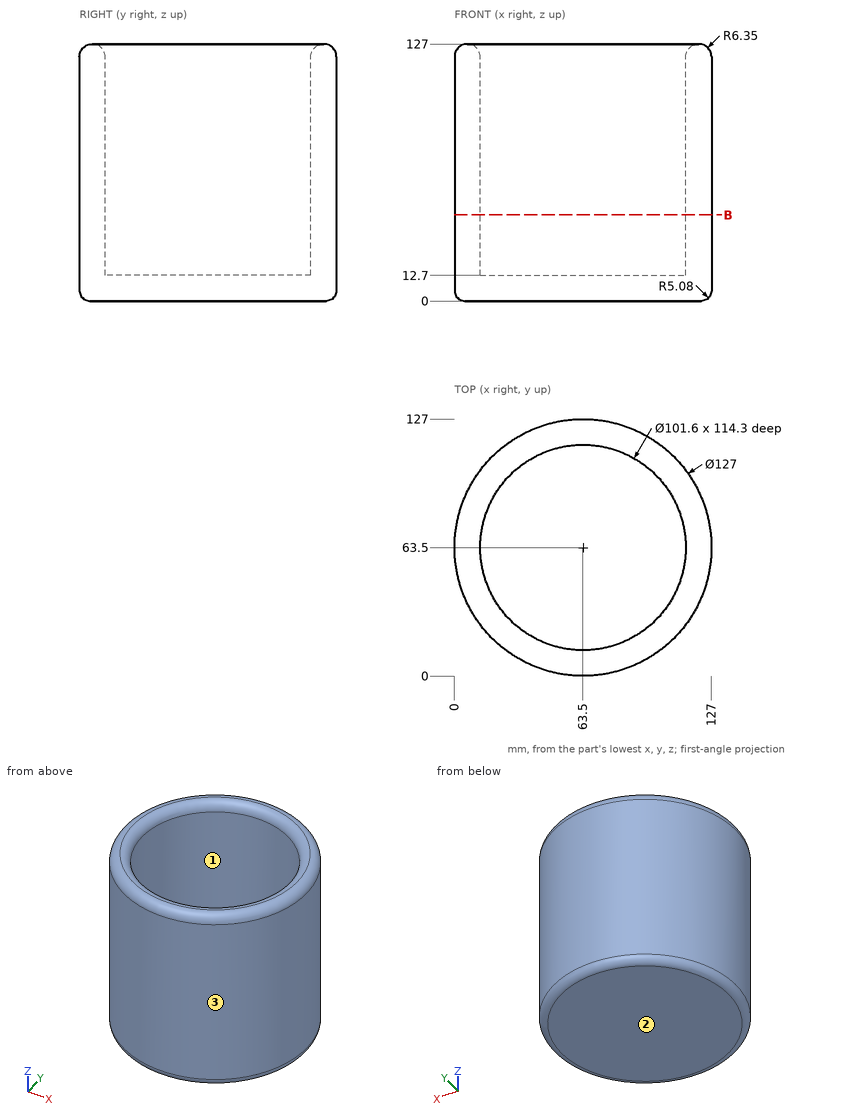
Here's the drawing with two shaded views (mm, measured from the low corner). I have some questions. Round coordinates to 2 decimals unless told otherwise and drop trailing zeros. Loops run counter-clockwise (first coordinate to the right, second up) from the corner with the lowest first, then second, coordinate; pieces in that order, holes last.
Item 1: Please list where these lines run through material, in increasing order: L1, parallel to Y at x = 64.5, z = 72; L2, parallel to X at y = 63, z = 39; L3, parallel to Z at x = 26.5, y = 55.
Item 2: If we mould it in two halves opening along X, with no side actions, what happens to the marked faces 1, 2 and 3? For each: +X half, -X half, draft (parallel to the pull), parting line (faces both ways), or undercut.
Item 3: Will these pins go through, and if not, where does the flat tip stop? pin 1 Ø1 at (y, z) = (32, 67) entering from +X; pin 2 Ø3 at (x, z) = (80.5, 85) entering from -Y; pin 3 Ø8 at (x, y) = (81.5, 45) entering from +Z.
Item 4: Suppose I cut it at B-B, the plane z = 42.5. Write out the boundary of the cut face in (x, y), then the cut area to 3 significant figures.
Reported:
1. L1: y = 0.01 to 12.71, 114.29 to 126.99
1. L2: x = 0 to 12.7, 114.3 to 127
1. L3: z = 0 to 12.7
2. face 1: undercut
2. face 2: draft
2. face 3: parting line
3. pin 1: stops at x = 118.92
3. pin 2: stops at y = 1.92
3. pin 3: stops at z = 12.7
4. outline: circle Ø127 at (63.5, 63.5); hole circle Ø101.6 at (63.5, 63.5)
4. area: 4,560 mm2
